Job drawing, mm, ordinate dimensions from the low corner. One solid piece. Give positions to 0.01 mm unless a question says otherwise; leave off trailing zeros. Order: outer loops, then holes, each group sorted by start corner. A loop starts at its lowest first (then second) coordinate and runs counter-clockwise, first axis right, second up. Notation, with made-up numbers: M 0.5,38.25 L 30.5,38.25 A25 ccw 30.5,73.25 Z; hole C 48.5,-15.75 d9. An arc over 180 degrees is marked long. One line per question, with ' | ' between items.
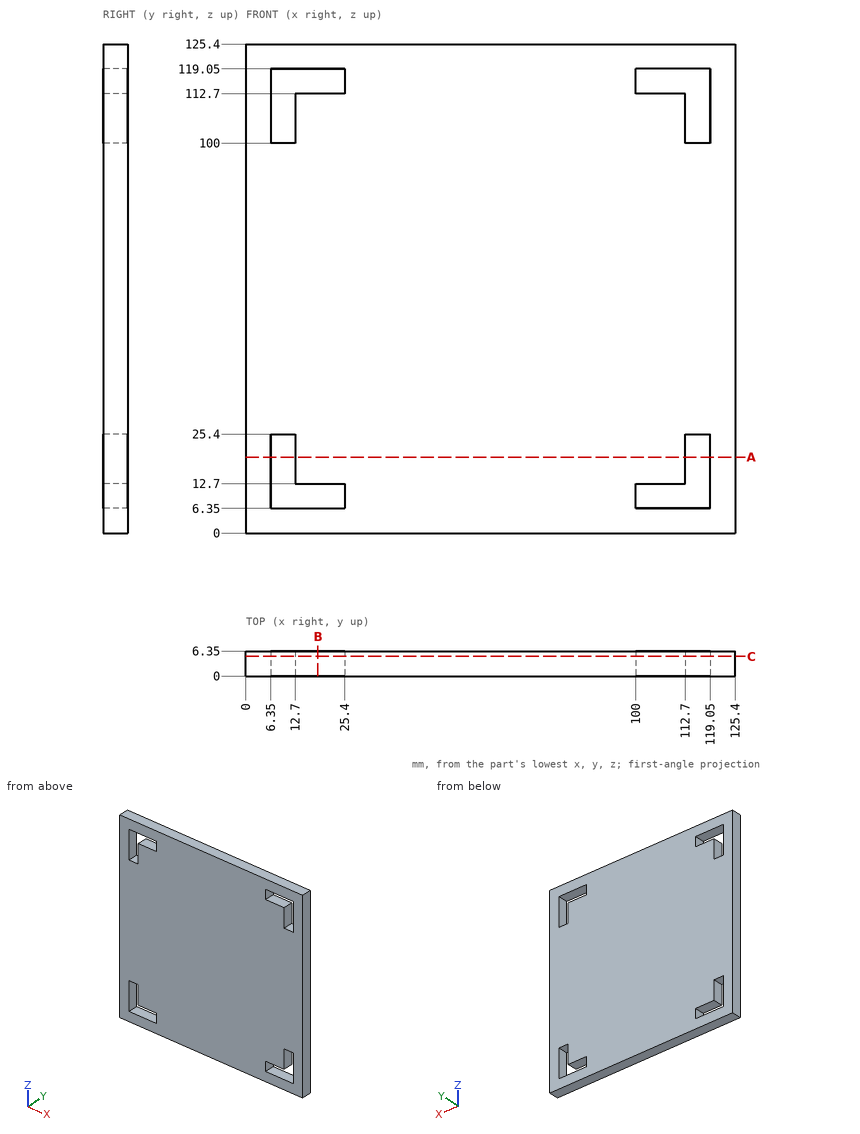
1. Probe L1, parallel to Z at x = 18.5, y = 3. List the from-to ranges inside material, lowest first. Write a range as from..to.
Worked out:
L1: z = 0..6.35, 12.7..112.7, 119.05..125.4
2. Slice it at A-A on z = 19.5. Give the cut face in (x, y), then the cut area to 3 significant figures.
Worked out:
outline: M 0,0 L 6.35,0 L 6.35,6.35 L 0,6.35 Z; M 12.7,0 L 112.7,0 L 112.7,6.35 L 12.7,6.35 Z; M 119.05,0 L 125.4,0 L 125.4,6.35 L 119.05,6.35 Z | area: 716 mm2
3. Slice it at B-B on x = 18.5. Give the cut face in (y, z), then the cut area to 3 significant figures.
Worked out:
outline: M 0,0 L 6.35,0 L 6.35,6.35 L 0,6.35 Z; M 0,12.7 L 6.35,12.7 L 6.35,112.7 L 0,112.7 Z; M 0,119.05 L 6.35,119.05 L 6.35,125.4 L 0,125.4 Z | area: 716 mm2
4. Slice it at C-C on y = 5. Give the cut face in (x, z), then the cut area to 3 significant figures.
Worked out:
outline: M 0,0 L 125.4,0 L 125.4,125.4 L 0,125.4 Z; hole M 6.35,6.35 L 25.4,6.35 L 25.4,12.7 L 12.7,12.7 L 12.7,25.4 L 6.35,25.4 Z; hole M 6.35,100 L 12.7,100 L 12.7,112.7 L 25.4,112.7 L 25.4,119.05 L 6.35,119.05 Z; hole M 100,6.35 L 119.05,6.35 L 119.05,25.4 L 112.7,25.4 L 112.7,12.7 L 100,12.7 Z; hole M 100,112.7 L 112.7,112.7 L 112.7,100 L 119.05,100 L 119.05,119.05 L 100,119.05 Z | area: 14,900 mm2
